Work out the finished part from the listing and answer in its coordinate system (mm). Face numbers are marked on the shaded views. A direction names the side the tool comes from. Round coordinates to 2 decimals unless told otherwise and drop trailing zeros. Write each loop counter-clockwise with the first axis right and the second up, starting at its lowest first coordinate (ties: lowest second). Pieces come first, ordered by that corner, then holes. Notation, with made-up numbers: (47.5, 28) - (59.5, 28) arc R21 cw to (59.5, 48) - close; hole circle Ø11 at (37, 59.25). An arc over 180 degrees is marked (long way). Answer as a JSON object with one key per item and string values.
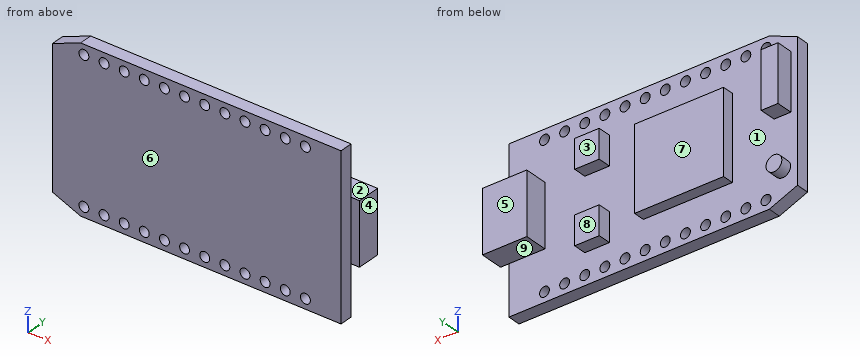
```python
from build123d import *

# Parameters (mm, degrees)
SKETCH1_W           = 36.55
SKETCH1_H           = 20.42
BOSS_EXTRUDE1_DEPTH = 1.64
CHAMFER1_SIZE       = 1.45
CHAMFER1_SIZE2      = 3.57
CHAMFER2_SIZE       = 3.57
CHAMFER2_SIZE2      = 1.45
SKETCH3_W           = 5.62
SKETCH3_H           = 7.85
BOSS_EXTRUDE2_DEPTH = 2.94
SKETCH4_W           = 3.11
SKETCH4_H           = 3.64
BOSS_EXTRUDE3_DEPTH = 1.65
SKETCH5_W           = 2.13
SKETCH5_H           = 7.16
BOSS_EXTRUDE4_DEPTH = 2.08
SKETCH6_W           = 11.27
SKETCH6_H           = 10.52
BOSS_EXTRUDE5_DEPTH = 1.43
SKETCH7_R           = 1
BOSS_EXTRUDE6_DEPTH = 1.43
SKETCH8_R           = 0.625
CUT_EXTRUDE1_DEPTH  = 2.64


with BuildPart() as part:
    # Sketch1 → Boss-Extrude1 (new body)
    with BuildSketch(Plane(origin=(0, 0, 0), x_dir=(1, 0, 0), z_dir=(0, 1, 0))):
        Rectangle(SKETCH1_W, SKETCH1_H)
    extrude(amount=BOSS_EXTRUDE1_DEPTH)

    # Chamfer1
    chamfer1_edges = [part.edges().sort_by_distance(p)[0] for p in [
        (-18.275, 0.82, 10.21),
    ]]
    chamfer1_side = [part.faces().sort_by_distance(p)[0] for p in [
        (-18.275, 0.82, 0),
    ]]
    chamfer(chamfer1_edges, length=CHAMFER1_SIZE, length2=CHAMFER1_SIZE2, reference=chamfer1_side[0])

    # Chamfer2
    chamfer2_edges = [part.edges().sort_by_distance(p)[0] for p in [
        (-18.275, 0.82, -10.21),
    ]]
    chamfer2_side = [part.faces().sort_by_distance(p)[0] for p in [
        (0, 0.82, -10.21),
    ]]
    chamfer(chamfer2_edges, length=CHAMFER2_SIZE, length2=CHAMFER2_SIZE2, reference=chamfer2_side[0])

    # Sketch3 → Boss-Extrude2 (add)
    with BuildSketch(Plane(origin=(0, 1.64, 0), x_dir=(1, 0, 0), z_dir=(0, 1, 0))):
        with Locations((16.525, 0)):
            Rectangle(SKETCH3_W, SKETCH3_H)
    extrude(amount=BOSS_EXTRUDE2_DEPTH)

    # Sketch4 → Boss-Extrude3 (add)
    with BuildSketch(Plane(origin=(0, 1.64, 0), x_dir=(1, 0, 0), z_dir=(0, 1, 0))):
        with Locations((7.1, 4.51)):
            Rectangle(SKETCH4_W, SKETCH4_H)
        with Locations((7.1, -4.51)):
            Rectangle(SKETCH4_W, SKETCH4_H)
    extrude(amount=BOSS_EXTRUDE3_DEPTH)

    # Sketch5 → Boss-Extrude4 (add)
    with BuildSketch(Plane(origin=(0, 1.64, 0), x_dir=(1, 0, 0), z_dir=(0, 1, 0))):
        with Locations((-16.37, -3.76)):
            Rectangle(SKETCH5_W, SKETCH5_H)
    extrude(amount=BOSS_EXTRUDE4_DEPTH)

    # Sketch6 → Boss-Extrude5 (add)
    with BuildSketch(Plane(origin=(0, 1.64, 0), x_dir=(1, 0, 0), z_dir=(0, 1, 0))):
        with Locations((-4.39, 0)):
            Rectangle(SKETCH6_W, SKETCH6_H)
    extrude(amount=BOSS_EXTRUDE5_DEPTH)

    # Sketch7 → Boss-Extrude6 (add)
    with BuildSketch(Plane(origin=(0, 1.64, 0), x_dir=(1, 0, 0), z_dir=(0, 1, 0))):
        with Locations((-16.405, 6.16)):
            Circle(SKETCH7_R)
    extrude(amount=BOSS_EXTRUDE6_DEPTH)

    # Sketch8 → Cut-Extrude1 (cut, through all)
    with BuildSketch(Plane(origin=(0, 1.64, 0), x_dir=(1, 0, 0), z_dir=(0, 1, 0))):
        with Locations((13.765, -8.96)):
            Circle(SKETCH8_R)
        with Locations((11.215, -8.96)):
            Circle(SKETCH8_R)
        with Locations((8.665, -8.96)):
            Circle(SKETCH8_R)
        with Locations((6.115, -8.96)):
            Circle(SKETCH8_R)
        with Locations((3.565, -8.96)):
            Circle(SKETCH8_R)
        with Locations((1.015, -8.96)):
            Circle(SKETCH8_R)
        with Locations((-1.535, -8.96)):
            Circle(SKETCH8_R)
        with Locations((-4.085, -8.96)):
            Circle(SKETCH8_R)
        with Locations((-6.635, -8.96)):
            Circle(SKETCH8_R)
        with Locations((-9.185, -8.96)):
            Circle(SKETCH8_R)
        with Locations((-11.735, -8.96)):
            Circle(SKETCH8_R)
        with Locations((-14.285, -8.96)):
            Circle(SKETCH8_R)
        with Locations((-14.285, 8.96)):
            Circle(SKETCH8_R)
        with Locations((-11.735, 8.96)):
            Circle(SKETCH8_R)
        with Locations((-9.185, 8.96)):
            Circle(SKETCH8_R)
        with Locations((3.565, 8.96)):
            Circle(SKETCH8_R)
        with Locations((-6.635, 8.96)):
            Circle(SKETCH8_R)
        with Locations((-4.085, 8.96)):
            Circle(SKETCH8_R)
        with Locations((-1.535, 8.96)):
            Circle(SKETCH8_R)
        with Locations((1.015, 8.96)):
            Circle(SKETCH8_R)
        with Locations((6.115, 8.96)):
            Circle(SKETCH8_R)
        with Locations((8.665, 8.96)):
            Circle(SKETCH8_R)
        with Locations((11.215, 8.96)):
            Circle(SKETCH8_R)
        with Locations((13.765, 8.96)):
            Circle(SKETCH8_R)
    extrude(amount=-CUT_EXTRUDE1_DEPTH, mode=Mode.SUBTRACT)


solid = part.part
```
Item 1: For the marked faces 5, 6, 7, 8 and 9, determine the directions among +Z, -Z, +X, -X, +Y, -Y from which every point of the face is accessible in a straight line to the end or side of a thin tool.
Results found:
{"face 5": "+Z, -Z, +X, -X, +Y", "face 6": "+Z, -Z, +X, -X, -Y", "face 7": "+Z, -Z, +Y", "face 8": "+Z, -Z, -X, +Y", "face 9": "-Z, +X, +Y"}
Item 2: Determine the mould class of the marked faces 1, 2, 3 and 4 for opening direction X: pulls with the +X half, pulls with the -X half, needs draft (parallel to the pull), parting line crosses it, or undercut.
Results found:
{"face 1": "undercut", "face 2": "needs draft", "face 3": "undercut", "face 4": "pulls with the +X half"}
Item 3: A cutting plane is placed at D-D (y = 0.35). Give the number of separate pieces and of enclosed holes in the cut face, and give its area (3 significant figures).
Results found:
{"separate pieces": "1", "enclosed holes": "24", "area": "712 mm²"}
Item 4: A cutting plane is placed at C-C (z = 1.25). Write down the section's boundary in (x, y) (3 decimals), and give its area (3 significant figures).
Results found:
{"outline": "(-18.275, 0) - (18.275, 0) - (18.275, 1.64) - (19.335, 1.64) - (19.335, 4.58) - (13.715, 4.58) - (13.715, 1.64) - (1.245, 1.64) - (1.245, 3.07) - (-10.025, 3.07) - (-10.025, 1.64) - (-15.305, 1.64) - (-15.305, 3.72) - (-17.435, 3.72) - (-17.435, 1.64) - (-18.275, 1.64) - close", "area": "97.0 mm²"}
Item 5: Each of these flat-tipped pins is pushed along its axis until it touches: P1, Ø0.6, axis at x = -17, y = 2, coming from the +Z side; P2, Ø1.1, axis at x = 1.015, z = -8.96, coming from the -Y side; P3, Ø0.5, axis at y = 2.5, z = 4.5, coming from the -X side (3 decimals); P4, Ø10, axis at x = -5.5, z = 2.5, coming from the +Y side. Where does it stop, or does it pass through?
Results found:
{"P1": "z = 7.34", "P2": "through", "P3": "x = -17.435", "P4": "y = 3.07"}
Item 6: A cutting plane is placed at A-A (y = 2.6). Write down the section's boundary in (x, z) (3 decimals), and give its area (3 significant figures).
Results found:
{"outline": "(-17.435, 0.18) - (-15.305, 0.18) - (-15.305, 7.34) - (-17.435, 7.34) - close; circle Ø2 at (-16.405, -6.16); (-10.025, -5.26) - (1.245, -5.26) - (1.245, 5.26) - (-10.025, 5.26) - close; (5.545, -6.33) - (8.655, -6.33) - (8.655, -2.69) - (5.545, -2.69) - close; (5.545, 2.69) - (8.655, 2.69) - (8.655, 6.33) - (5.545, 6.33) - close; (13.715, -3.925) - (19.335, -3.925) - (19.335, 3.925) - (13.715, 3.925) - close", "area": "204 mm²"}
Item 7: A cutting plane is placed at B-B (x = 11). Write down the section's boundary in (y, z), and give its area (3 significant figures).
Results found:
{"outline": "(0, -10.21) - (1.64, -10.21) - (1.64, -9.55) - (0, -9.55) - close; (0, -8.37) - (1.64, -8.37) - (1.64, 8.37) - (0, 8.37) - close; (0, 9.55) - (1.64, 9.55) - (1.64, 10.21) - (0, 10.21) - close", "area": "29.6 mm²"}
Item 8: Consider line 1 along Y through (x, z) = (10.5, -9.5); line 2 along X through (y, z) = (0.2, 6.5) (3 decimals); line 3 along Z through (x, y) = (9, 1.05). Determine where each line is inside the solid, lowest interval first.
Results found:
{"line 1": "0 to 1.64", "line 2": "-18.275 to 18.275", "line 3": "-10.21 to -9.49, -8.43 to 8.43, 9.49 to 10.21"}
